CAD build for the part. Positions are in the model's coordinates, mm. Face numbers are marked on the shaded views. Give positions to 0.01 mm unless a question says otherwise; leave off trailing zeros. Order: outer loops, then holes, each group sorted by start corner. A loop starts at its lowest first (then second) coordinate and runs counter-clockwise, first axis right, second up. Notation, with made-up numbers: (34.5, 50) -> (46.5, 50) arc R28 ccw to (46.5, 83) -> close; hole circle Ø2 at (-21.5, 63). An arc over 180 degrees is marked (long way). Use one line per item in the form item = value. Start each with the question number.
1) Cut at A-A, the plane z = -11.5. Give the cut face in (x, y).
2) Drop flat-ended pins along their axis: P1, Ø1.5, axis at x = -3, z = 2, coming from the -Y side; P2, Ø1.1, axis at x = -6.02, z = 11.1, coming from the +Y side; P3, Ø3, axis at x = -7, y = 3, coming from the -Z side (3 decimals); P4, Ø2.5, axis at x = -6, y = 4, coming from the +Z side. Give the stop position or say it passes through.
3) Cut at D-D, the plane z = 8. Give the cut face in (x, y), and give its area (3 significant figures).
4) Mould opens along X. For the marked faces 1, 2, 3 and 4 say: pulls with the +X half, pulls with the -X half, needs draft (parallel to the pull), parting line crosses it, or undercut.
5) Probe line 1 (Y direction, x = -7.16, z = -9); line 2 (Y direction, x = -7, z = 3.5); line 3 (X direction, y = 3.25, z = -14). List the from-to ranges inside material, lowest first.
6) Cut at C-C, the plane x = 10.5. Give the cut face in (y, z).
7) Cut at B-B, the plane y = -0.25. Give the cut face in (x, z) (3 decimals).
from build123d import *

# Parameters (mm, degrees)
SKETCH1_W           = 25.4
SKETCH1_H           = 25.4
BOSS_EXTRUDE1_DEPTH = 0.8001
SKETCH2_R           = 0.635
CUT_EXTRUDE1_DEPTH  = 1.6002
SKETCH3_W           = 6
SKETCH3_H           = 14.605
BOSS_EXTRUDE2_DEPTH = 5
SKETCH4_R           = 2.5
BOSS_EXTRUDE3_DEPTH = 2.3
SKETCH5_R           = 1.75
CUT_EXTRUDE4_DEPTH  = 15.905
CHAMFER1_SIZE       = 0.25
SKETCH6_R           = 0.9
SKETCH6_R_2         = 0.635
BOSS_EXTRUDE4_DEPTH = 0.01


with BuildPart() as part:
    # Sketch1 → Boss-Extrude1 (new body, symmetric)
    with BuildSketch(Plane(origin=(0, 0, 0), x_dir=(1, 0, 0), z_dir=(0, 1, 0))):
        Rectangle(SKETCH1_W, SKETCH1_H)
    extrude(amount=BOSS_EXTRUDE1_DEPTH, both=True)

    # Sketch2 → Cut-Extrude1 (cut)
    with BuildSketch(Plane(origin=(0, 0.8001, 0), x_dir=(1, 0, 0), z_dir=(0, 1, 0))):
        with Locations((-11.0998, -11.0998)):
            Circle(SKETCH2_R)
        with Locations((-8.5598, -11.0998)):
            Circle(SKETCH2_R)
        with Locations((-6.0198, -11.0998)):
            Circle(SKETCH2_R)
        with Locations((1.6002, -11.0998)):
            Circle(SKETCH2_R)
        with Locations((4.1402, -11.0998)):
            Circle(SKETCH2_R)
    extrude(amount=-CUT_EXTRUDE1_DEPTH, mode=Mode.SUBTRACT)

    # Sketch3 → Boss-Extrude2 (add)
    with BuildSketch(Plane(origin=(0, 0.8001, 0), x_dir=(1, 0, 0), z_dir=(0, 1, 0))):
        with Locations((-7.16, 6.0025)):
            Rectangle(SKETCH3_W, SKETCH3_H)
    extrude(amount=BOSS_EXTRUDE2_DEPTH)

    # Sketch4 → Boss-Extrude3 (add)
    with BuildSketch(Plane(origin=(0, 0, -13.305), x_dir=(-1, 0, 0), z_dir=(0, 0, -1))):
        with Locations((7.16, 3.3001)):
            Circle(SKETCH4_R)
    extrude(amount=BOSS_EXTRUDE3_DEPTH)

    # Sketch5 → Cut-Extrude4 (cut)
    with BuildSketch(Plane(origin=(0, 0, -15.605), x_dir=(-1, 0, 0), z_dir=(0, 0, -1))):
        with Locations((7.16, 3.3001)):
            Circle(SKETCH5_R)
    extrude(amount=-CUT_EXTRUDE4_DEPTH, mode=Mode.SUBTRACT)

    # Chamfer1
    chamfer1_edges = [part.edges().sort_by_distance(p)[0] for p in [
        (-4.66, 3.3001, -15.605),
    ]]
    chamfer(chamfer1_edges, length=CHAMFER1_SIZE)

    # Sketch6 → Boss-Extrude4 (add)
    with BuildSketch(Plane(origin=(0, 0.8001, 0), x_dir=(1, 0, 0), z_dir=(0, 1, 0))):
        with Locations((-11.0998, -11.0998)):
            Circle(SKETCH6_R)
        with Locations((-11.0998, -11.0998)):
            Circle(SKETCH6_R_2, mode=Mode.SUBTRACT)
        with Locations((-8.5598, -11.0998)):
            Circle(SKETCH6_R)
        with Locations((-8.5598, -11.0998)):
            Circle(SKETCH6_R_2, mode=Mode.SUBTRACT)
        with Locations((-6.0198, -11.0998)):
            Circle(SKETCH6_R)
        with Locations((-6.0198, -11.0998)):
            Circle(SKETCH6_R_2, mode=Mode.SUBTRACT)
        with Locations((1.6002, -11.0998)):
            Circle(SKETCH6_R)
        with Locations((1.6002, -11.0998)):
            Circle(SKETCH6_R_2, mode=Mode.SUBTRACT)
        with Locations((4.1402, -11.0998)):
            Circle(SKETCH6_R)
        with Locations((4.1402, -11.0998)):
            Circle(SKETCH6_R_2, mode=Mode.SUBTRACT)
    boss_extrude4 = extrude(amount=BOSS_EXTRUDE4_DEPTH)

    # Mirror1: Boss-Extrude4 across plane
    add(boss_extrude4.mirror(Plane.ZX))


solid = part.part
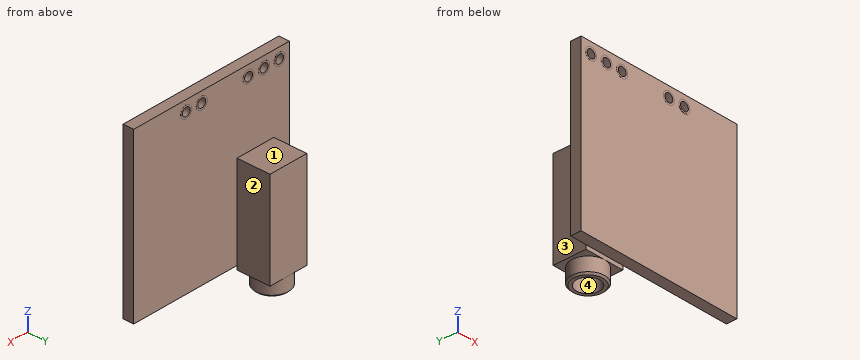
Result:
q1.outline = (-12.7, -0.8) -> (12.7, -0.8) -> (12.7, 0.8) -> (-4.16, 0.8) -> (-4.16, 5.8) -> (-10.16, 5.8) -> (-10.16, 0.8) -> (-12.7, 0.8) -> close; hole circle Ø3.5 at (-7.16, 3.3)
q2.P1 = -0.8
q2.P2 = through
q2.P3 = -15.605
q2.P4 = 1.3
q3.outline = (-12.7, -0.8) -> (12.7, -0.8) -> (12.7, 0.8) -> (-12.7, 0.8) -> close
q3.area = 40.6 mm²
q4.face_1 = needs draft
q4.face_2 = pulls with the +X half
q4.face_3 = pulls with the -X half
q4.face_4 = undercut
q5.line_1 = -0.8 to 1.55, 5.05 to 5.8
q5.line_2 = -0.8 to 0.8
q5.line_3 = -9.66 to -8.91, -5.41 to -4.66
q6.outline = (-0.8, -12.7) -> (0.8, -12.7) -> (0.8, 12.7) -> (-0.8, 12.7) -> close
q7.outline = (-12.7, -12.7) -> (12.7, -12.7) -> (12.7, 12.7) -> (-12.7, 12.7) -> close; hole circle Ø1.27 at (-11.1, 11.1); hole circle Ø1.27 at (-8.56, 11.1); hole circle Ø1.27 at (-6.02, 11.1); hole circle Ø1.27 at (1.6, 11.1); hole circle Ø1.27 at (4.14, 11.1)
